Check sheet for the modelled part. Datum: model origin and axes. Units: mm. Round coordinates to 2 decimals unless told otherwise and drop trailing zeros. Order: outer loops, then holes, each group sorted by start corner. A loop starts at its lowest first (then second) coordinate and runs counter-clockwise, first axis right, second up.
Q1. Depth check by flat-ended pin: P1, Ø8, axis at x = -394.5, z = 0, coming from the -Y side; P2, Ø1, axis at x = 85.5, y = 5.5, coming from the +Z side; P3, Ø4, axis at x = -323.5, y = -11, coming from the -Z side. Enter the tip coordinate at first touch or a pass-through.
Q2. Cross-section at A-A on x = -272.5. Record the cut outline in (y, z).
Q3. Scan lines: probe 1 along X at (y, z) = (0, -47.5); probe 2 along X at (y, z) = (-4.5, -51.5); probe 3 along Z at (x, y) = (52.5, 0). Record each from-to range of solid material in increasing order.
Q4. Mould release check, pull along X, two halves, no side actions. Record for faces 1 (the flat face through (-541.35, -3.82, -106.87)), 2 (the flat face through (541.35, -3.82, -106.87)), 3 (the cylindrical face through (-476.22, -5.42, -26.04)): +X half, -X half, draft (parallel to the pull), parting line (faces both ways), or undercut.
from build123d import *

# Parameters (mm, degrees)
F1_R   = 25
F1_R_2 = 22.5
F6_D   = 8.8


with BuildPart() as f2:
    # F2: sweep along a path in F0
    with BuildLine(Plane.XZ) as f2_path:
        Line((0, 24.8682312667), (-338, 24.8682312667))
        ThreePointArc((-338, 24.8682312667), (-364.3925829493, 22.0501921499), (-389.5951606003, 13.723136311))
        Line((-389.5951606003, 13.723136311), (-560.8329377868, -63.8759852319))
    # F1 (on Right) → F2 (sweep)
    with BuildSketch(Plane.YZ):
        Circle(F1_R)
        Circle(F1_R_2, mode=Mode.SUBTRACT)
    sweep(path=f2_path.line)

    # F3: F2 across plane


with BuildPart() as f2_1:
    add(f2.part)
    add(f2.part.mirror(Plane.YZ))

    # F6 (through all)
    with Locations(Plane.XY.offset(25)):
        with Locations((0, 0)):
            Hole(F6_D / 2)


solid = f2_1.part
Results found:
1. P1: stops at y = -22.74
1. P2: stops at z = 24.49
1. P3: stops at z = -23.32
2. outline: circle Ø50 at (0, 0); hole circle Ø45 at (0, 0)
3. probe 1: x = -525.02 to -518.96, -409.94 to -403.88, 403.88 to 409.94, 518.96 to 525.02
3. probe 2: x = -532.85 to -526.68, -419.86 to -413.7, 413.7 to 419.86, 526.68 to 532.85
3. probe 3: z = -25 to -22.5, 22.5 to 25
4. face 1: -X half
4. face 2: +X half
4. face 3: undercut
